Verification items for the finished model (mm, model axes). Face numbers are marked on the shaded views. A direction names the side the tool comes from. Coordinates: 2 decimals unless noted, no trailing zeros. Loops run counter-clockwise (first coordinate to the right, second up) from the corner with the lowest first, then second, coordinate; pieces in that order, holes last. Notation, with made-up numbers: (50, 89.25) -> (85, 89.25) arc R25 ccw to (85, 118.25) -> close; hole circle Ø5 at (34, 15). An arc over 180 degrees is marked (long way). Answer as a JSON object with one key per item and string values. Group by question number.
Q1. Scan lines: L1, parallel to X at y = 16.5, z = -2; L2, parallel to Y at x = 12.5, z = -0.75 (3 decimals); L3, parallel to Y at x = 12.7, z = -0.85 (3 decimals). Record each from-to range of solid material in increasing order.
Q2. Cross-section at C-C on y = 22. Record the boundary of the cut face in (x, z) (3 decimals), and give its area (3 significant figures).
Q3. Release check for a two-part mould opening along Y. For the marked faces 3, 4 and 5 record: released by +Y, released by -Y, zero draft, split by the parting line, or undercut.
Q4. Set-up check for the marked faces 1 and 2: record each of +Z, -Z, +X, -X, +Y, -Y from which the full face is reachable in a straight line by a thin tool's end or side.
Q5. Gauge pin test, flat ends, axial feed: pin 1 Ø5 at (x, y) = (45.72, 8.509) entering from +Z; pin 2 Ø10.5 at (x, y) = (12.7, 16.637) entering from -Z; pin 3 Ø5 at (x, y) = (5.08, 8.509) entering from -Z (3 decimals). Record the tip position at first contact, or that the pin passes through.
Q6. Cross-section at B-B on x = 41. Record the boundary of the cut face in (y, z) (3 decimals), and give its area (3 significant figures).
Q7. Cross-section at A-A on z = -9.25. Record the boundary of the cut face in (x, y) (3 decimals), and give its area (3 significant figures).
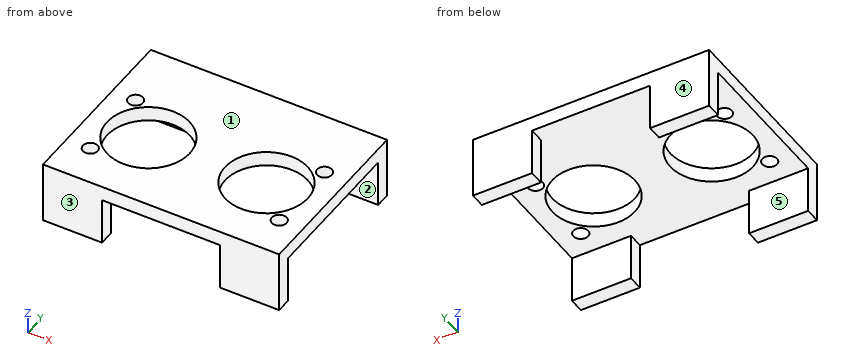
Autodesk Inventor part; units mm, degrees
ref_plane "YZ Plane" through (0, 0, 0) normal (1, 0, 0) x (0, 1, 0)
ref_plane "XZ Plane" through (0, 0, 0) normal (0, 1, 0) x (-1, 0, 0)
ref_plane "XY Plane" through (0, 0, 0) normal (0, 0, 1) x (1, 0, 0)
sketch "Sketch1" plane through (0, 0, 0) normal (1, 0, 0) x (0, 1, 0)
  line L0 (0, 0) -> (35.56, 0)
  line L1 (35.56, -3.175) -> (3.175, -3.175)
  line L2 (3.175, -3.175) -> (3.175, -13.335)
  line L3 (3.175, -13.335) -> (0, -13.335)
  line L4 (0, -13.335) -> (0, 0)
  line L5 (35.56, 0) -> (38.735, 0)
  line L6 (38.735, 0) -> (38.735, -13.335)
  line L7 (38.735, -13.335) -> (35.56, -13.335)
  line L8 (35.56, -13.335) -> (35.56, -3.175)
  dimension "d0" = 3.175
  dimension "d1" = 35.56
  dimension "d33" = 13.335
  dimension "d34" = 3.175
  dimension "d48" = 90
  dimension "d49" = 13.335
  dimension "d50" = 3.175
  dimension "d51" = 10.16
extrude "Extrusion1" add sketch "Sketch1" along normal blind 50.8
sketch "Sketch3" plane through (0, 0, 0) normal (0, 0, 1) x (1, 0, 0)
  line L0 (0, 35.56) -> (50.8, 35.56)
  line L1 (25.4, 35.56) -> (25.4, 3.175) construction
  line L2 (0, 3.175) -> (50.8, 3.175)
  circle A0 centre (12.7, 16.637) radius 8.89
  circle A1 centre (38.1, 16.637) radius 8.89
  line L3 (0, 0) -> (0, 35.56)
  line L4 (0, 27.305) -> (50.8, 27.305) construction
  line L5 (0, 5.969) -> (52.4314, 5.969) construction
  line L6 (2.54, 27.305) -> (2.54, 5.969) construction
  line L7 (48.26, 27.305) -> (48.26, 5.969) construction
  circle A2 centre (5.08, 8.509) radius 1.5875
  circle A3 centre (45.72, 24.765) radius 1.5875
  circle A4 centre (5.08, 24.765) radius 1.5875
  circle A5 centre (45.72, 8.509) radius 1.5875
  dimension "d7" = 17.78
  dimension "d8" = 12.7
  dimension "d13" = 10.668
  dimension "d14" = 10.668
  dimension "d15" = 10.16
  dimension "d16" = 10.16
  dimension "d17" = 3.175
  dimension "d19" = 2.54
  dimension "d20" = 3.175
  dimension "d21" = 2.54
  dimension "d25" = 2.54
  dimension "d26" = 2.54
  dimension "d38" = 3.175
  dimension "d39" = 2.54
  dimension "d40" = 2.54
  dimension "d41" = 3.175
  dimension "d42" = 2.54
  dimension "d43" = 2.54
  dimension "d53" = 2.794
extrude "Extrusion2" cut sketch "Sketch3" against normal through all
sketch "Sketch5" plane through (0, 38.735, 0) normal (0, 1, 0) x (1, 0, 0)
  line L0 (0, 0) -> (50.8, 0) construction
  line L1 (0, 3.175) -> (50.8, 3.175) construction
  line L2 (12.7, 3.175) -> (12.7, 13.335)
  line L3 (0, 13.335) -> (50.8, 13.335)
  line L4 (38.1, 3.175) -> (38.1, 13.335)
  line L5 (0, 0) -> (0, 13.335)
  line L6 (12.7, 3.175) -> (38.1, 3.175)
  line L7 (12.7, 13.335) -> (38.1, 13.335)
  dimension "d44" = 25.4
  dimension "d45" = 12.7
extrude "Extrusion4" cut sketch "Sketch5" against normal through all
equation "\"d49\" = d33"
equation "\"d50\" = d0"
properties part number "ping_bracket"
Computed values:
{
 "1": {"L1": "x = 0 to 3.81, 21.59 to 29.21, 46.99 to 50.8", "L2": "y = 0 to 7.749, 25.525 to 38.735", "L3": "y = 0 to 7.747, 25.527 to 38.735"},
 "2": {"outline": "(0, -3.175) -> (5.61, -3.175) -> (5.61, 0) -> (0, 0) -> close; (19.79, -3.175) -> (31.01, -3.175) -> (31.01, 0) -> (19.79, 0) -> close; (45.19, -3.175) -> (50.8, -3.175) -> (50.8, 0) -> (45.19, 0) -> close", "area": "71.2 mm²"},
 "3": {"face 3": "released by -Y", "face 4": "released by +Y", "face 5": "undercut"},
 "4": {"face 1": "+Z, +X, -X, +Y, -Y", "face 2": "-Z, +X, -X"},
 "5": {"pin 1": "stops at z = 0", "pin 2": "passes through", "pin 3": "stops at z = -3.175"},
 "6": {"outline": "(0, -13.335) -> (3.175, -13.335) -> (3.175, -3.175) -> (8.233, -3.175) -> (8.233, 0) -> (0, 0) -> close; (25.041, -3.175) -> (35.56, -3.175) -> (35.56, -13.335) -> (38.735, -13.335) -> (38.735, 0) -> (25.041, 0) -> close", "area": "134 mm²"},
 "7": {"outline": "(0, 0) -> (12.7, 0) -> (12.7, 3.175) -> (0, 3.175) -> close; (0, 35.56) -> (12.7, 35.56) -> (12.7, 38.735) -> (0, 38.735) -> close; (38.1, 0) -> (50.8, 0) -> (50.8, 3.175) -> (38.1, 3.175) -> close; (38.1, 35.56) -> (50.8, 35.56) -> (50.8, 38.735) -> (38.1, 38.735) -> close", "area": "161 mm²"}
}
